Geometry check sheet. Reference: drawing and pictorial views, mm from the part's lowest x, y, z. Coordinates: 2 decimals unless noted, no trailing zeros. Loops run counter-clockwise (first coordinate to the right, second up) from the corner with the lowest first, then second, coordinate; pieces in that order, holes last. Notation, with made-up numbers: (73, 71) - (87, 71) arc R20 cw to (87, 89) - close; hole circle Ø10 at (-36.75, 87). An arc over 180 degrees is marked (long way). Use a Markdown table: item, result. Add a question column.
1) Thickness scan on line 1 (Y direction, x = 116, z = 1.7); line 2 (Y direction, x = 12.5, z = 2.25); line 3 (Y direction, x = 86.5, z = 0.1). Record the ranges inside material, lowest first.
2) Sectioned sample at C-C, the plane y = 28. Enter the section's corners in (x, z).
3) Go/stop test with flat-tipped pins: P1, Ø1, axis at x = 60.5, z = 0.5, coming from the -Y side; P2, Ø4.5, axis at x = 116, y = 8, coming from the -Z side (3 decimals); P3, Ø0.9, axis at y = 24, z = 1.5, coming from the -X side. Record where each tip stops, or that it passes through.
4) Sectioned sample at B-B, the plane z = 1. Enter the section's corners in (x, y).
5) Sectioned sample at D-D, the plane x = 37.5. Enter the section's corners in (y, z), then the cut area to 4 significant figures.
6) Sectioned sample at A-A, the plane x = 116. Enter the section's corners in (y, z).
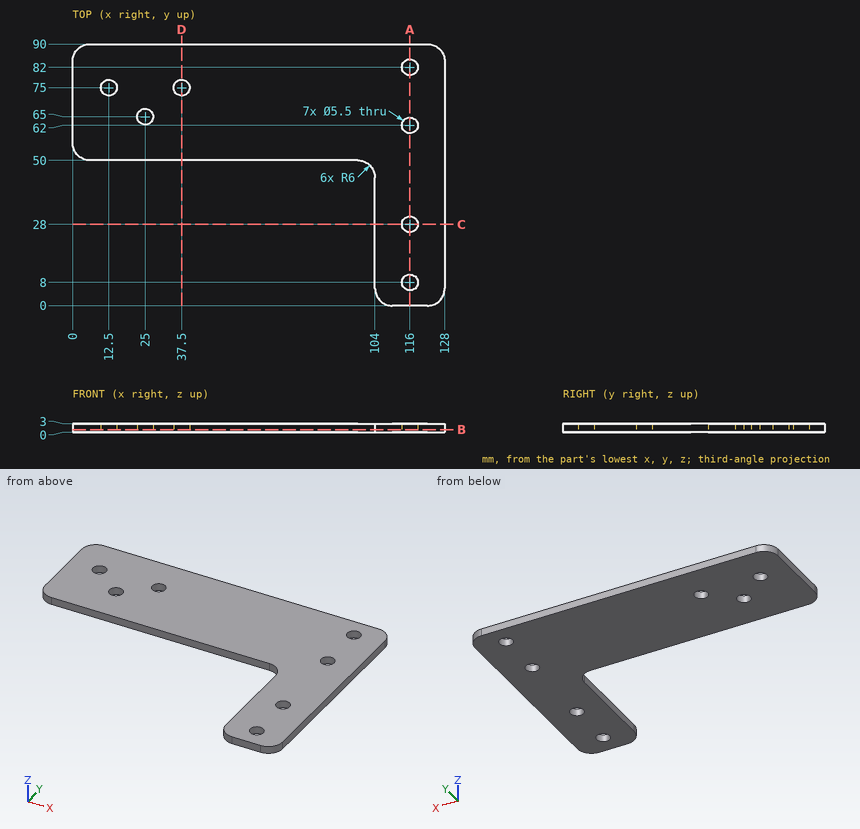
Solved:
| question | item | result |
|---|---|---|
| 1 | line 1 | y = 0 to 5.25, 10.75 to 25.25, 30.75 to 59.25, 64.75 to 79.25, 84.75 to 90 |
| 1 | line 2 | y = 50 to 72.25, 77.75 to 90 |
| 1 | line 3 | y = 50 to 90 |
| 2 | outline | (104, 0) - (113.25, 0) - (113.25, 3) - (104, 3) - close; (118.75, 0) - (128, 0) - (128, 3) - (118.75, 3) - close |
| 3 | P1 | stops at y = 50 |
| 3 | P2 | passes through |
| 3 | P3 | stops at x = 104 |
| 4 | outline | (0, 56) arc R6 ccw to (6, 50) - (98, 50) arc R6 cw to (104, 44) - (104, 6) arc R6 ccw to (110, 0) - (122, 0) arc R6 ccw to (128, 6) - (128, 84) arc R6 ccw to (122, 90) - (6, 90) arc R6 ccw to (0, 84) - close; hole circle Ø5.5 at (12.5, 75); hole circle Ø5.5 at (25, 65); hole circle Ø5.5 at (37.5, 75); hole circle Ø5.5 at (116, 8); hole circle Ø5.5 at (116, 28); hole circle Ø5.5 at (116, 62); hole circle Ø5.5 at (116, 82) |
| 5 | outline | (50, 0) - (72.25, 0) - (72.25, 3) - (50, 3) - close; (77.75, 0) - (90, 0) - (90, 3) - (77.75, 3) - close |
| 5 | area | 103.5 mm2 |
| 6 | outline | (0, 0) - (5.25, 0) - (5.25, 3) - (0, 3) - close; (10.75, 0) - (25.25, 0) - (25.25, 3) - (10.75, 3) - close; (30.75, 0) - (59.25, 0) - (59.25, 3) - (30.75, 3) - close; (64.75, 0) - (79.25, 0) - (79.25, 3) - (64.75, 3) - close; (84.75, 0) - (90, 0) - (90, 3) - (84.75, 3) - close |
